Read the model definition and answer for the solid it produces. Units are mm, in the model's axes. A direction names the side the tool comes from. Give positions to 0.01 mm unless a question says otherwise; leave off trailing zeros. Loops run counter-clockwise (first coordinate to the right, second up) from the corner with the lowest first, then second, coordinate; pieces in that order, holes last. Notation, with made-up numbers: (58, 59.25) - (82, 59.25) arc R21 cw to (82, 84.25) - close; hole circle Ø2 at (2.5, -15). An arc over 180 degrees is marked (long way). Put each result on its own line as item: value. Start each with the question number.
1. A cutting plane is placed at C-C, the plane z = -1. Determine the outline of the cut face in (x, y), plus the area to 3 significant figures.
2. A cutting plane is placed at A-A, the plane x = 0. Determine the outline of the cut face in (y, z).
3. A cutting plane is placed at B-B, the plane y = 2.75. Determine the outline of the cut face in (x, z).
4. A cutting plane is placed at D-D, the plane z = -14. Determine the outline of the cut face in (x, y), plus the area to 3 significant figures.
5. For a pull along X with two mould halves and no side action, classify faces 1 (the flat face through (4, 2, -9)), 2 (the flat face through (3, 4, -12)), 3 (the cylindrical face through (-0.1, 1, 3.5)) as released by +X, released by -X, zero draft, split by the parting line, or undercut.
6. For faces 4 (the flat face through (2.872, 2.965, -7.782)), 5 (the flat face through (-4, 2, -9)), 6 (the cylindrical face through (1.34, -1.57, -16.39)), 7 (the cylindrical face through (0.1, 1, -3.5)), determine the directions among +Z, -Z, +X, -X, +Y, -Y from which every point of the face is accessible in a straight line to the end or side of a thin tool.
7. Given pin 1 Ø1.7 at (x, y) = (-0.5, 2.5) entering from +Z; pin 2 Ø1.5 at (x, y) = (1, 0) entering from -Z, each flat-ended and moving along its own axis, determine where each tip first touches the part or whether it passes through.
8. Consider L1, parallel to Z at x = 0, y = 2.6; L2, parallel to X at y = 2.3, z = -18.5; L3, parallel to X at y = 1.4, z = 0. Determine where each line is inside the solid, lowest interval first. Write a range as from..to.
Autodesk Inventor part; units mm, degrees
ref_plane "YZ Plane" through (0, 0, 0) normal (1, 0, 0) x (0, 1, 0)
ref_plane "XZ Plane" through (0, 0, 0) normal (0, 1, 0) x (-1, 0, 0)
ref_plane "XY Plane" through (0, 0, 0) normal (0, 0, 1) x (1, 0, 0)
sketch "Эскиз1" plane through (0, 0, 0) normal (0, 1, 0) x (-1, 0, 0)
  circle A0 centre (0, 0) radius 4
  dimension "d0" = 8
extrude "Выдавливание1" add sketch "Эскиз1" along normal blind 4
sketch "Эскиз5" plane through (0, 4, 0) normal (0, 1, 0) x (1, 0, 0)
  circle A0 centre (0, 0) radius 4
  line L0 (-4, 0) -> (4, 0)
  line L1 (4, 0) -> (4, 18.5)
  line L2 (4, 18.5) -> (-4, 18.5)
  line L3 (-4, 18.5) -> (-4, 0)
  circle A1 centre (0, 0) radius 4
  point P0 (4, 0)
  dimension "d27" = 18.5
extrude "Выдавливание4" add sketch "Эскиз5" against normal blind 4 contours A0 L3 L2 L1
sketch "Эскиз9" plane through (0, 4, 0) normal (0, -1, 0) x (1, 0, 0)
  circle A0 centre (0, 0) radius 3.5
  line L0 (3.5, 0) -> (-3.5, 0)
  line L1 (3.5, 0) -> (2.25, -15.5)
  line L2 (-3.5, 0) -> (-2.25, -15.5)
  line L3 (2.25, -15.5) -> (-2.25, -15.5)
  point P0 (0, -15.5)
  point P1 (-3.4548, -0.5609)
  point P2 (3.4548, -0.5609)
  dimension "d43" = 7
  dimension "d44" = 4.5
  dimension "d45" = 15.5
extrude "Выдавливание7" cut sketch "Эскиз9" along normal blind 2.1
sketch "Эскиз10" plane through (0, 1.9, 0) normal (0, 1, 0) x (1, 0, 0)
  line L0 (2.25, 15.5) -> (3.4548, 0.5609)
  line L1 (-2.25, 15.5) -> (2.25, 15.5)
  line L2 (-3.4548, 0.5609) -> (-2.25, 15.5)
  arc A0 (-3.4548, 0.5609) -> (3.4548, 0.5609) centre (0, 0) ccw
  arc A1 (-3.4548, 0.5609) -> (3.4548, 0.5609) centre (0, 0) ccw
  circle A2 centre (0, 0) radius 3.5
  point P0 (3.4548, 0.5609)
extrude "Выдавливание8" cut sketch "Эскиз10" against normal through all contours A0 A2
sketch "Эскиз6" plane through (0, 4, 0) normal (0, 1, 0) x (1, 0, 0)
  line L0 (-4, 18.5) -> (4, 18.5)
  circle A0 centre (0, 18.5) radius 4
  point P0 (0, 0)
  dimension "d30" = 8
extrude "Выдавливание5" add sketch "Эскиз6" against normal blind 6.8
sketch "Эскиз7" plane through (0, -2.8, -18.5) normal (0, -1, 0) x (1, 0, 0)
  arc A0 (-4, 0) -> (4, 0) centre (0, 0) ccw
  arc A1 (4, 0) -> (-4, 0) centre (0, 0) ccw
  circle A2 centre (0, 0) radius 2.5
  point P0 (0, 18.5)
  point P1 (3.35, -2.1857)
  point P2 (-3.35, -2.1857)
  dimension "d33" = 5
extrude "Выдавливание6" cut sketch "Эскиз7" against normal blind 2.5 contours A2
sketch "Эскиз8" plane through (0, 4, 0) normal (0, 1, 0) x (1, 0, 0)
  circle A0 centre (0, 18.5) radius 2.5
  point P0 (0, 0)
hole "Отверстие2" at (0, 4, -18.5) direction (0, -1, 0) diameter 3 end through all
sketch "Эскиз11" plane through (0, 4, 0) normal (0, 1, 0) x (1, 0, 0)
  line L0 (-3.4548, 0.5609) -> (-2.2735, 15.2089)
  line L1 (2.2735, 15.2089) -> (3.4548, 0.5609)
  line L2 (-2.2735, 15.2089) -> (2.2735, 15.2089)
  arc A0 (-2.2735, 15.2089) -> (2.2735, 15.2089) centre (0, 18.5) ccw
  line L3 (-3.4548, 0.5609) -> (-2.2735, 15.2089)
  arc A1 (3.4548, 0.5609) -> (-3.4548, 0.5609) centre (0, 0) ccw
  line L4 (2.2735, 15.2089) -> (3.4548, 0.5609)
extrude "Выдавливание9" cut sketch "Эскиз11" against normal up to surface (2.1 mm away)
properties part number "Поворотный рычаг для сервы"
Return value:
1. outline: (-4, 0) - (-3.35, 0) - (-3.35, 1.9) - (-3.42, 1.9) - (-3.42, 4) - (-4, 4) - close; (3.35, 0) - (4, 0) - (4, 4) - (3.42, 4) - (3.42, 1.9) - (3.35, 1.9) - close
1. area: 4.89 mm2
2. outline: (-2.8, -22.5) - (4, -22.5) - (4, -20) - (-0.3, -20) - (-0.3, -21) - (-2.8, -21) - close; (-2.8, -16) - (-0.3, -16) - (-0.3, -17) - (4, -17) - (4, -15.21) - (1.9, -15.21) - (1.9, -3.5) - (0, -3.5) - (0, -14.5) - (-2.8, -14.5) - close; (0, 3.5) - (4, 3.5) - (4, 4) - (0, 4) - close
3. outline: (-4, -18.5) arc R4 ccw to (4, -18.5) - (4, 0) arc R4 ccw to (-4, 0) - close; hole (-3.45, -0.56) - (-2.27, -15.21) - (2.27, -15.21) - (3.45, -0.56) arc R3.5 ccw (long way) to start; hole circle Ø3 at (0, -18.5)
4. outline: (-4, 0) - (4, 0) - (4, 4) - (2.37, 4) - (2.37, 1.9) - (-2.37, 1.9) - (-2.37, 4) - (-4, 4) - close
4. area: 22.0 mm2
5. face 1: released by +X
5. face 2: zero draft
5. face 3: undercut
6. face 4: +Y
6. face 5: +Z, -Z, -X, +Y, -Y
6. face 6: -Y
6. face 7: +Y, -Y
7. pin 1: stops at z = 4
7. pin 2: stops at z = -22.49
8. L1: z = -22.5..-20, -17..-15.21, 3.5..4
8. L2: x = -4..-1.5, 1.5..4
8. L3: x = -4..-3.5, 3.5..4
